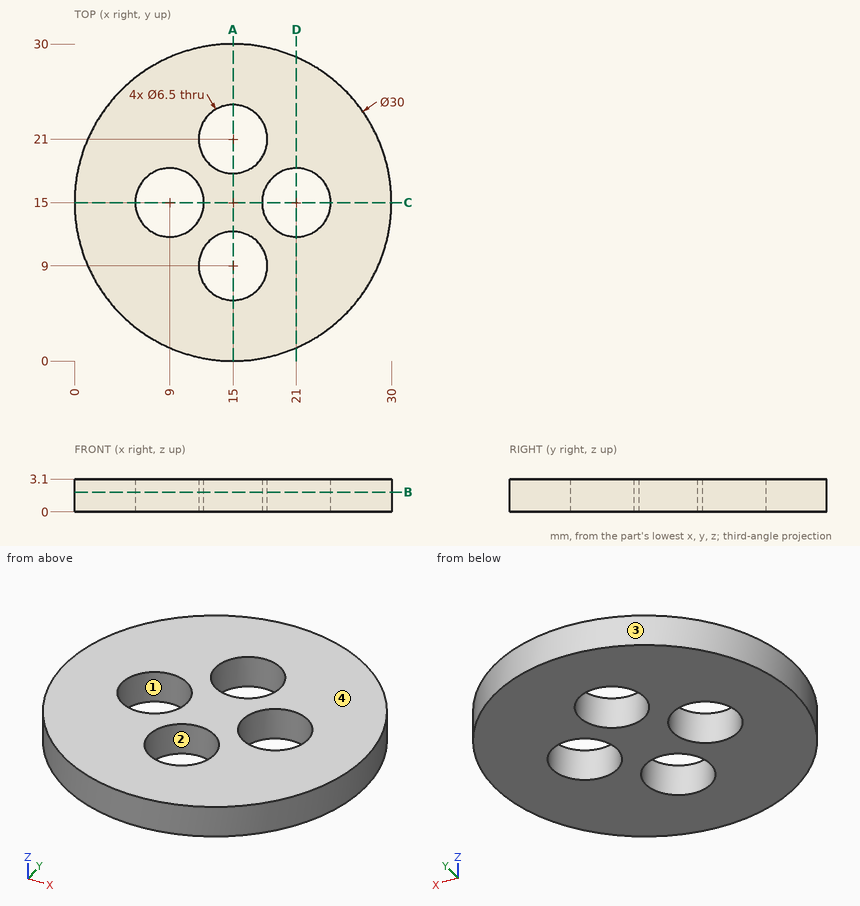
Here's the drawing with two shaded views (mm, measured from the low corner). I have some questions. Round coordinates to 2 decimals unless told otherwise and drop trailing zeros. Loops run counter-clockwise (first coordinate to the right, second up) from the corner with the lowest first, then second, coordinate; pieces in that order, holes last. Notation, with made-up numbers: M 47.5,22.5 L 60.5,22.5 A6 ccw 60.5,32.5 Z; hole C 15,67.5 d8. An arc over 180 degrees is marked long. Answer as CSV lines item,"result".
1) If I drill on probe 1 along Y at (x, z) = (15, 2.3); probe 2 along X at (y, z) = (13.75, 2.35); probe 3 along X at (y, z) = (15.25, 2.55), over which ranges is the centre line in solid material (lowest first)?
From the geometry:
probe 1,"0 to 5.75, 12.25 to 17.75, 24.25 to 30"
probe 2,"0.05 to 6, 12 to 18, 24 to 29.95"
probe 3,"0 to 5.76, 12.24 to 17.76, 24.24 to 30"
2) Imagine slicing it at B-B on z = 1.85. List the corners of the cut face in (x, y) for me, and give its area (3 significant figures).
From the geometry:
outline,"C 15,15 d30; hole C 9,15 d6.5; hole C 15,9 d6.5; hole C 15,21 d6.5; hole C 21,15 d6.5"
area,"574 mm^2"
3) We'd pull the mould along Y, two halves only. Please class the marked faces 1, 2, 3 and 4: released by +Y, released by -Y, zero draft, split by the parting line, or undercut.
From the geometry:
face 1,"undercut"
face 2,"undercut"
face 3,"split by the parting line"
face 4,"zero draft"
4) Imagine slicing it at D-D on x = 21. List the corners of the cut face in (y, z) for me, and give its area (3 significant figures).
From the geometry:
outline,"M 1.25,0 L 11.75,0 L 11.75,3.1 L 1.25,3.1 Z; M 18.25,0 L 28.75,0 L 28.75,3.1 L 18.25,3.1 Z"
area,"65.1 mm^2"
5) Imagine slicing it at A-A on x = 15. List the corners of the cut face in (y, z) for me, and give its area (3 significant figures).
From the geometry:
outline,"M 0,0 L 5.75,0 L 5.75,3.1 L 0,3.1 Z; M 12.25,0 L 17.75,0 L 17.75,3.1 L 12.25,3.1 Z; M 24.25,0 L 30,0 L 30,3.1 L 24.25,3.1 Z"
area,"52.7 mm^2"
